Design review of the part built by this model. Coordinates are the model's own, in mm. A direction names the side the tool comes from. Give positions to 0.01 mm unless a question says otherwise; leave off trailing zeros. Write each loop counter-clockwise with the first axis right and the second up, starting at its lowest first coordinate (ties: lowest second). Pieces come first, ordered by that corner, then holes. Notation, with made-up numbers: (6.5, -31.75) -> (64.5, -31.75) arc R21 ccw to (64.5, -0.75) -> close; hole circle Ø4 at (-5, 4.5). An arc over 180 degrees is marked (long way). Answer as a JSON object with one key per item and string values.
```python
from build123d import *

# Parameters (mm, degrees)
CYLINDER938_R          = 1.25
CYLINDER938_DEPTH      = 10
CYLINDER938_ROLL_ANGLE = 90
CYLINDER939_R          = 1.25
CYLINDER939_DEPTH      = 20
CYLINDER939_ROLL_ANGLE = 90
CYLINDER937_R          = 5.2
CYLINDER937_DEPTH      = 10
BOX555_W               = 16
BOX555_H               = 20
BOX555_DEPTH           = 10
CUT690_ROLL_ANGLE      = 90


with BuildPart() as cylinder1081:
    # Cylinder938 → Cylinder938 (new body)
    with BuildSketch(Plane.XY):
        Circle(CYLINDER938_R)
    extrude(amount=CYLINDER938_DEPTH)


with BuildPart() as cylinder1081_1:
    # Cylinder938 roll: moved
    add(cylinder1081.part.rotate(Axis((0, 0, 0), (1, 0, 0)), CYLINDER938_ROLL_ANGLE))


with BuildPart() as cylinder1081_2:
    # Cylinder938 placement: moved
    add(cylinder1081_1.part.moved(Location((0, 10, 2))))


with BuildPart() as fusion587:
    # Cylinder939 → Cylinder939 (new body)
    with BuildSketch(Plane.XY):
        Circle(CYLINDER939_R)
    extrude(amount=CYLINDER939_DEPTH)


with BuildPart() as fusion587_1:
    # Cylinder939 roll: moved
    add(fusion587.part.rotate(Axis((0, 0, 0), (1, 0, 0)), CYLINDER939_ROLL_ANGLE))


with BuildPart() as fusion587_2:
    # Cylinder939 placement: moved
    add(fusion587_1.part.moved(Location((0, 10, 7.5))))

    # Fusion587: union Cylinder1081
    add(cylinder1081_2.part)


with BuildPart() as cylinder1080:
    # Cylinder937 → Cylinder937 (new body)
    with BuildSketch(Plane.XY):
        Circle(CYLINDER937_R)
    extrude(amount=CYLINDER937_DEPTH)


with BuildPart() as servo_shaft_coupler_holes:
    # Box555 → Box555 (new body)
    with BuildSketch(Plane(origin=(-8, -10, 0), x_dir=(1, 0, 0), z_dir=(0, 0, 1))):
        with Locations((8, 10)):
            Rectangle(BOX555_W, BOX555_H)
    extrude(amount=BOX555_DEPTH)

    # Cut689: cut Cylinder1080
    add(cylinder1080.part, mode=Mode.SUBTRACT)

    # Cut690: cut Fusion587
    add(fusion587_2.part, mode=Mode.SUBTRACT)


with BuildPart() as servo_shaft_coupler_holes_1:
    # Cut690 roll: moved
    add(servo_shaft_coupler_holes.part.rotate(Axis((0, 0, 0), (1, 0, 0)), CUT690_ROLL_ANGLE))


with BuildPart() as servo_shaft_coupler_holes_2:
    # Cut690 placement: moved
    add(servo_shaft_coupler_holes_1.part.moved(Location((37, 73, -11))))


solid = servo_shaft_coupler_holes_2.part
```
(1) The part is to be moulded in two halves that separate along X. For faces 3 (the flat face through (45, 68, -11)), 4 (the cylindrical face through (36.84, 64.26, -18.49)), 5 (the flat face through (29, 68, -11)), 6 (the flat face through (31.6, 63, -10.9)), say which applies: +X half, -X half, draft (parallel to the pull), parting line (faces both ways), or undercut.
Here are the results:
{"face 3": "+X half", "face 4": "undercut", "face 5": "-X half", "face 6": "draft"}
(2) We need section A-A, the plane x = 37. State the section outline as (y, z) points, then the cut area to 3 significant figures.
Here are the results:
{"outline": "(63, -21) -> (64.25, -21) -> (64.25, -16.2) -> (63, -16.2) -> close; (63, -5.8) -> (64.25, -5.8) -> (64.25, -1) -> (63, -1) -> close; (66.75, -21) -> (73, -21) -> (73, -16.2) -> (66.75, -16.2) -> close; (66.75, -5.8) -> (69.75, -5.8) -> (69.75, -1) -> (66.75, -1) -> close; (72.25, -5.8) -> (73, -5.8) -> (73, -1) -> (72.25, -1) -> close", "area": "60.0 mm²"}
(3) Clearance check with a flat-ended pin moving along its axis: pin 1 (2 mm diameter, centred on x = 37, y = 71, fed in from +Z). State where the tip first meets the part, or that it passes through.
Here are the results:
{"pin 1": "stops at z = -16.1"}
(4) For faces 1 (the cylindrical face through (36.84, 69.76, -3.44)), 2 (the flat face through (31.6, 73, -10.9)), list the 3-axis set-ups (+Z, -Z, +X, -X, +Y, -Y) from which the entire face can be reached by the end or side of a thin tool; tool diameter is ignored.
Here are the results:
{"face 1": "+Z", "face 2": "+Z, -Z, +X, -X, +Y"}
(5) For line 1 along X through (y, z) = (65.5, -4.55); line 2 along Y through (x, z) = (37, -1.95); line 3 along Z through (x, y) = (37, 67.75), list the stretches that pass through material, from the lowest coordinate up.
Here are the results:
{"line 1": "x = 29 to 35.75, 38.25 to 45", "line 2": "y = 63 to 64.25, 66.75 to 69.75, 72.25 to 73", "line 3": "z = -21 to -16.2, -5.8 to -1"}
(6) We need section B-B, the plane z = -11. State the section outline as (x, y) points.
Here are the results:
{"outline": "(29, 63) -> (31.8, 63) -> (31.8, 73) -> (29, 73) -> close; (42.2, 63) -> (45, 63) -> (45, 73) -> (42.2, 73) -> close"}
(7) We need section D-D, the plane x = 39. State the section outline as (y, z) points.
Here are the results:
{"outline": "(63, -21) -> (73, -21) -> (73, -15.8) -> (63, -15.8) -> close; (63, -6.2) -> (73, -6.2) -> (73, -1) -> (63, -1) -> close"}
(8) We need section C-C, the plane y = 65.5. State the section outline as (x, z) points.
Here are the results:
{"outline": "(29, -21) -> (35.75, -21) -> (35.75, -16.05) arc R5.2 cw to (35.75, -5.95) -> (35.75, -1) -> (29, -1) -> close; (38.25, -21) -> (45, -21) -> (45, -1) -> (38.25, -1) -> (38.25, -5.95) arc R5.2 cw to (38.25, -16.05) -> close"}
